Input: dimensioned drawing with shaded views. Units: mm. Origin: part minimum x, y, z. A direction names the side the tool comes from. Coordinates: 2 decimals unless noted, no trailing zeros. Order: outer loops, then holes, each group sorted by start corner. A loop starts at its lowest first (then second) coordinate and runs counter-clockwise, first axis right, second up.
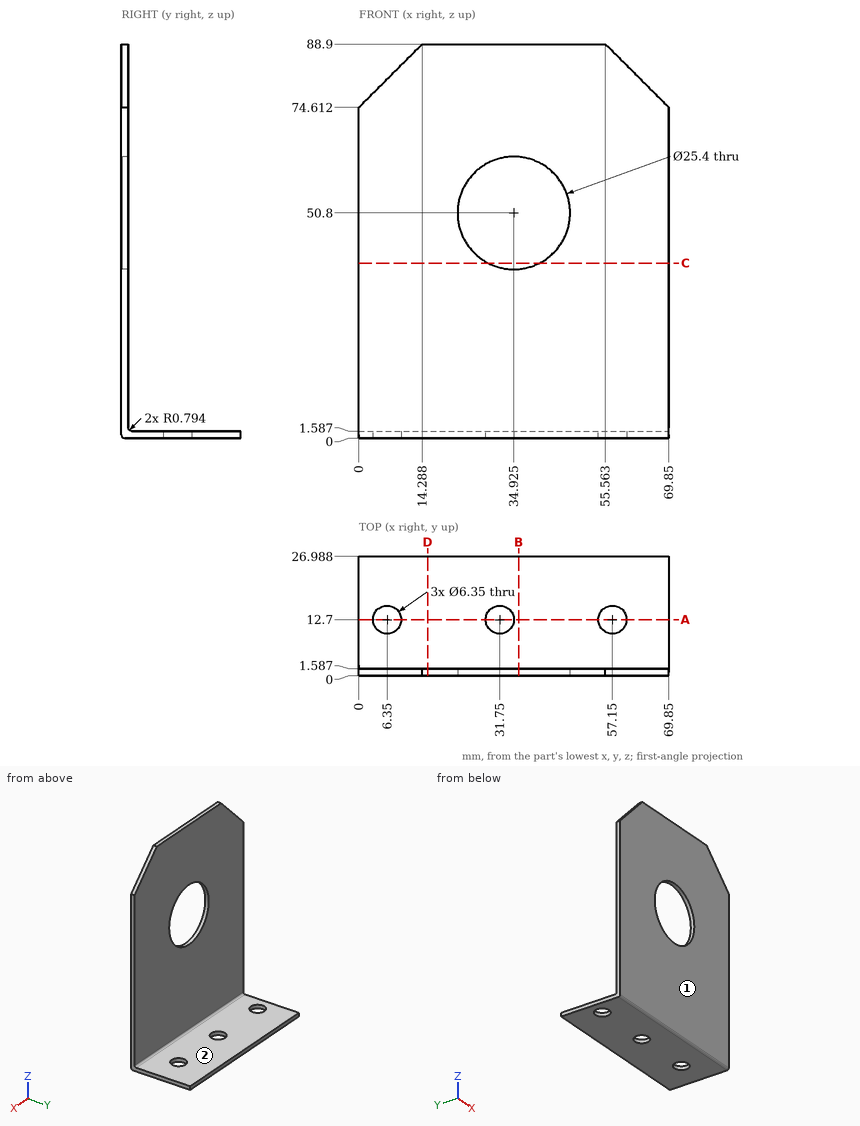
1. Access query for the marked faces 1 and 2. Directions: +Z, -Z, +X, -X, +Y, -Y. A direction counts if a zero-diameter tool reaches every point of the face in a straight line with its end or side. Return the directions, or none.
2. Contact query for flat-ended pins moving along their axis: P1, Ø4, axis at x = 57.15, y = 12.7, coming from the +Z side; P2, Ø12, axis at x = 42.5, y = 18, coming from the +Z side; P3, Ø6, axis at x = 54.5, z = 79.5, coming from the +Y side. Output: stop coordinate, or through.
3. Section query D-D, the plane x = 15.5. Output: boundary loops of the cut face in (y, z).
4. Material intervals for line 1 along Y through (x, z) = (6.35, 1) (1 decimal); line 2 along Y through (x, z) = (57.5, 80.5), sorted ascending.
5. Section query C-C, the plane z = 39.5. Output: boundary loops of the cut face in (x, y).
6. Section query B-B, the plane x = 36. Output: boundary loops of the cut face in (y, z) (1 decimal), plus the area to 3 significant figures.
7. Section query A-A, the plane y = 12.7. Count the separate pieces of the cut face and the enclosed holes in it.
Answer key:
1. face 1: +Z, -Z, +X, -X, -Y
1. face 2: +Z, +X, -X, +Y
2. P1: passes through
2. P2: stops at z = 1.59
2. P3: stops at y = 1.59
3. outline: (0, 0.79) arc R0.79 ccw to (0.79, 0) - (26.99, 0) - (26.99, 1.59) - (2.38, 1.59) arc R0.79 cw to (1.59, 2.38) - (1.59, 88.9) - (0, 88.9) - close
4. line 1: y = 0 to 9.5, 15.9 to 27
4. line 2: y = 0 to 1.59
5. outline: (0, 0) - (29.13, 0) - (29.13, 1.59) - (0, 1.59) - close; (40.72, 0) - (69.85, 0) - (69.85, 1.59) - (40.72, 1.59) - close
6. outline: (0, 0.8) arc R0.8 ccw to (0.8, 0) - (27, 0) - (27, 1.6) - (2.4, 1.6) arc R0.8 cw to (1.6, 2.4) - (1.6, 38.1) - (0, 38.1) - close; (0, 63.5) - (1.6, 63.5) - (1.6, 88.9) - (0, 88.9) - close
6. area: 141 mm2
7. separate pieces: 4
7. enclosed holes: 0
